```python
from build123d import *

# Parameters (mm, degrees)
F0_W           = 50
F0_H           = 50
F1_DEPTH       = 5
F2_W           = 45
F2_H           = 5
F3_DEPTH       = 45
F4_R           = 25
F5_R           = 2
F9_D           = 3.1
F9_DEPTH       = 20
F9_TIP         = 0.9313339595
F9_ON_F6_D     = 3.1
F9_ON_F6_DEPTH = 20
F9_ON_F6_TIP   = 0.9313339595
F9_ON_F8_D     = 3.1
F9_ON_F8_DEPTH = 20
F9_ON_F8_TIP   = 0.9313339595


with BuildPart() as f1:
    # F0 (on Top) → F1 (new body)
    with BuildSketch(Plane.XY):
        Rectangle(F0_W, F0_H)
    extrude(amount=F1_DEPTH)

    # F2 (on face) → F3 (join)
    with BuildSketch(Plane.XY.offset(5)):
        Polygon((-20, 25), (-25, 25), (-25, -25), (-20, -25), (-20, 20), align=None)
        with Locations((2.5, 22.5)):
            Rectangle(F2_W, F2_H)
    extrude(amount=F3_DEPTH)

    # F4
    f4_edges = [f1.edges().sort_by_distance(p)[0] for p in [
        (25, 22.5, 50),
        (-22.5, -25, 50),
        (25, -25, 2.5),
    ]]
    fillet(f4_edges, radius=F4_R)

    # F5
    f5_edges = [f1.edges().sort_by_distance(p)[0] for p in [
        (-12.5, -25, 0),
        (17.67767, -17.67767, 0),
        (-25, 0, 0),
        (25, 12.5, 0),
        (0, 25, 0),
        (-25, 12.5, 50),
        (-25, -17.67767, 42.67767),
        (-25, 25, 25),
        (-25, -25, 12.5),
        (25, 25, 12.5),
        (17.67767, 25, 42.67767),
        (-12.5, 25, 50),
    ]]
    fillet(f5_edges, radius=F5_R)

    # F9
    with Locations(Plane.YZ.offset(-20)):
        with Locations((-2.5, 27.5)):
            Hole(F9_D / 2, depth=F9_DEPTH)
            with Locations((0, 0, -(F9_DEPTH + F9_TIP / 2))):  # 118° drill point
                Cone(0, F9_D / 2, F9_TIP, mode=Mode.SUBTRACT)

    # F9 on F6
    with Locations(Plane.XY.offset(5)):
        with Locations((2.5, -2.5)):
            Hole(F9_ON_F6_D / 2, depth=F9_ON_F6_DEPTH)
            with Locations((0, 0, -(F9_ON_F6_DEPTH + F9_ON_F6_TIP / 2))):  # 118° drill point
                Cone(0, F9_ON_F6_D / 2, F9_ON_F6_TIP, mode=Mode.SUBTRACT)

    # F9 on F8
    with Locations(Plane.XZ.offset(-20)):
        with Locations((2.5, 27.5)):
            Hole(F9_ON_F8_D / 2, depth=F9_ON_F8_DEPTH)
            with Locations((0, 0, -(F9_ON_F8_DEPTH + F9_ON_F8_TIP / 2))):  # 118° drill point
                Cone(0, F9_ON_F8_D / 2, F9_ON_F8_TIP, mode=Mode.SUBTRACT)


solid = f1.part
```
CAD build for the part. Positions are in the model's coordinates, mm. A direction names the side the tool comes from. Round coordinates to 2 decimals unless told otherwise and drop trailing zeros. Write each loop counter-clockwise with the first axis right and the second up, starting at its lowest first coordinate (ties: lowest second). Pieces come first, ordered by that corner, then holes. Notation, with made-up numbers: (2.25, 6) - (34.25, 6) arc R8 cw to (34.25, 13) - close; hole circle Ø4 at (11.25, 63.5). An arc over 180 degrees is marked (long way). Write item = value, one per line. Start each with the question number.
Q1. Band-saw the part on C-C (z = 27.5). Count the separate pieces of the cut face and the enclosed holes in it, then the cut area to 3 significant figures.
Q2. Probe L1, parallel to Y at x = 10, z = 39; L2, parallel to Z at x = -1, y = -11; L3, parallel to X at y = -2.5, z = 12.5. List the from-to ranges inside material, lowest first. Write a range as from..to.
Q3. Band-saw the part on A-A (x = -9.5). Give the cut face in (y, z), then the cut area to 3 significant figures.
Q4. Band-saw the part on B-B (y = 9). Give the cut face in (x, z), then the cut area to 3 significant figures.
Q5. Which spindle directions (+Z, -Z, +X, -X, +Y, -Y) get a long thin tool onto all of the face, cutting with end or side? Do faces 1 (the flat face through (-20, -3, 22)), 2 (the cylindrical face through (-21.479, -17.871, 42.482)). Say none if no direction does.
Q6. Mould opens along X. For faces 3 (the flat face through (-16, -25, 4)), 4 (the cylindrical face through (24.43, 11.66, 0.6)), 5 (the cylindrical face through (2.702, 22.535, 29.037)) say: pulls with the +X half, pulls with the -X half, needs draft (parallel to the pull), parting line crosses it, or undercut.
Q7. Drop flat-ended pins along their axis: pin 1 (12 mm diameter, centred on x = -8, z = 25.5, fed in from -Y); pin 2 (22.5 mm diameter, centred on x = 0.5, y = 5, fed in from +Z); pin 3 (22.5 mm diameter, centred on y = 5, z = 26.5, fed in from +X); pin 4 (6 mm diameter, centred on x = 1.5, y = -15, fed in from -Z). Give the stop position or say it passes through.
Answers below:
q1.separate_pieces = 3
q1.enclosed_holes = 0
q1.area = 440 mm2
q2.L1 = 20..25
q2.L2 = 0..5
q2.L3 = -25..-20
q3.outline = (-25, 2) arc R2 ccw to (-23, 0) - (23, 0) arc R2 ccw to (25, 2) - (25, 48) arc R2 ccw to (23, 50) - (20, 50) - (20, 5) - (-25, 5) - close
q3.area = 472 mm2
q4.outline = (-25, 2) arc R2 ccw to (-23, 0) - (23, 0) arc R2 ccw to (25, 2) - (25, 5) - (-20, 5) - (-20, 50) - (-23, 50) arc R2 ccw to (-25, 48) - close
q4.area = 472 mm2
q5.face_1 = +Z, +X, -Y
q5.face_2 = +Z, +X, -X, -Y
q6.face_3 = needs draft
q6.face_4 = pulls with the +X half
q6.face_5 = undercut
q7.pin_1 = 20
q7.pin_2 = 5
q7.pin_3 = -20
q7.pin_4 = 0
